```python
from build123d import *

# Parameters (mm, degrees)
AUFSATZ_LINEAR_AUSTRAGEN1_DEPTH      = 20
SCHNITT_LINEAR_AUSTRAGEN1_DEPTH      = 84.102346537
SKIZZE3_R                            = 3.15
SCHNITT_LINEAR_AUSTRAGEN2_DEPTH      = 84.102346537
SCHNITT_LINEAR_AUSTRAGEN3_DEPTH      = 2
SKIZZE5_R                            = 0.75
SCHNITT_LINEAR_AUSTRAGEN4_DEPTH      = 2
SKIZZE6_W                            = 35.5
SKIZZE6_H                            = 6.955295524
AUFSATZ_LINEAR_AUSTRAGEN2_DEPTH      = 20
SKIZZE7_W                            = 7.611739691
SKIZZE7_H                            = 53.192525908
AUFSATZ_LINEAR_AUSTRAGEN3_DEPTH      = 20
SKIZZE8_W                            = 7
SKIZZE8_H                            = 20
AUFSATZ_LINEAR_AUSTRAGEN4_DEPTH      = 27.7
SCHNITT_LINEAR_AUSTRAGEN5_DEPTH      = 26.48
SCHNITT_LINEAR_AUSTRAGEN6_DEPTH      = 6
SCHNITT_LINEAR_AUSTRAGEN6_DEPTH_BACK = 26.48
SKIZZE10_R                           = 1.75
SKIZZE11_R                           = 3
AUFSATZ_LINEAR_AUSTRAGEN5_DEPTH      = 4
SKIZZE12_W                           = 4.692525908
SKIZZE12_H                           = 20
SCHNITT_LINEAR_AUSTRAGEN7_DEPTH      = 130.77615571


with BuildPart() as part:
    # Skizze1 → Aufsatz-Linear austragen1 (new body)
    with BuildSketch(Plane(origin=(0, 0, 0), x_dir=(1, 0, 0), z_dir=(0, 1, 0))):
        with BuildLine():
            Line((0, 59), (0, 0))
            Line((0, 0), (3, 0))
            Line((3, 0), (3, 51.3))
            ThreePointArc((3, 51.3), (4.376598128, 54.623401872), (7.7, 56))
            Line((7.7, 56), (47.3, 56))
            ThreePointArc((47.3, 56), (50.623401872, 54.623401872), (52, 51.3))
            Line((52, 51.3), (52, 0))
            Line((52, 0), (55, 0))
            Line((55, 0), (55, 54.3))
            ThreePointArc((55, 54.3), (53.623401872, 57.623401872), (50.3, 59))
            Line((50.3, 59), (0, 59))
        make_face()
    extrude(amount=AUFSATZ_LINEAR_AUSTRAGEN1_DEPTH)

    # Skizze2 → Schnitt-Linear austragen1 (cut, through all)
    with BuildSketch(Plane(origin=(55, 0, 0), x_dir=(0, 0, -1), z_dir=(1, 0, 0))):
        with BuildLine():
            ThreePointArc((0, 10), (2.928932188, 17.071067812), (10, 20))
            Line((10, 20), (0, 20))
            Line((0, 20), (0, 10))
        make_face()
        with BuildLine():
            ThreePointArc((10, 0), (2.928932188, 2.928932188), (0, 10))
            Line((0, 10), (0, 0))
            Line((0, 0), (10, 0))
        make_face()
    extrude(amount=-SCHNITT_LINEAR_AUSTRAGEN1_DEPTH, mode=Mode.SUBTRACT)

    # Skizze3 → Schnitt-Linear austragen2 (cut, through all)
    with BuildSketch(Plane(origin=(55, 0, 0), x_dir=(0, 0, -1), z_dir=(1, 0, 0))):
        with Locations((10, 10)):
            Circle(SKIZZE3_R)
    extrude(amount=-SCHNITT_LINEAR_AUSTRAGEN2_DEPTH, mode=Mode.SUBTRACT)

    # Skizze4 → Schnitt-Linear austragen3 (cut)
    with BuildSketch(Plane.ZY.offset(-52)):
        with BuildLine():
            Line((-27.5, 7.5), (-12.823894492, 4.145461598))
            ThreePointArc((-12.823894492, 4.145461598), (-3.5, 10), (-12.823894492, 15.854538402))
            Line((-12.823894492, 15.854538402), (-27.5, 12.5))
            ThreePointArc((-27.5, 12.5), (-30, 10), (-27.5, 7.5))
        make_face()
    extrude(amount=-SCHNITT_LINEAR_AUSTRAGEN3_DEPTH, mode=Mode.SUBTRACT)

    # Skizze5 → Schnitt-Linear austragen4 (cut)
    with BuildSketch(Plane.ZY.offset(-54)):
        with Locations((-26.5, 10)):
            Circle(SKIZZE5_R)
        with Locations((-23.5, 10)):
            Circle(SKIZZE5_R)
        with Locations((-20.5, 10)):
            Circle(SKIZZE5_R)
        with Locations((-17.5, 10)):
            Circle(SKIZZE5_R)
    extrude(amount=-SCHNITT_LINEAR_AUSTRAGEN4_DEPTH, mode=Mode.SUBTRACT)

    # Skizze6 → Aufsatz-Linear austragen2 (add)
    with BuildSketch(Plane.XZ):
        with Locations((17.75, -62.477647762)):
            Rectangle(SKIZZE6_W, SKIZZE6_H)
    extrude(amount=-AUFSATZ_LINEAR_AUSTRAGEN2_DEPTH)

    # Skizze7 → Aufsatz-Linear austragen3 (add)
    with BuildSketch(Plane.XZ):
        with Locations((3.805869846, -92.551558478)):
            Rectangle(SKIZZE7_W, SKIZZE7_H)
    extrude(amount=-AUFSATZ_LINEAR_AUSTRAGEN3_DEPTH)

    # Skizze8 → Aufsatz-Linear austragen4 (add)
    with BuildSketch(Plane(origin=(7.611739691, 0, 0), x_dir=(0, 0, -1), z_dir=(1, 0, 0))):
        with Locations((110.955295524, 10)):
            Rectangle(SKIZZE8_W, SKIZZE8_H)
    extrude(amount=AUFSATZ_LINEAR_AUSTRAGEN4_DEPTH)

    # Skizze9 → Schnitt-Linear austragen5 (cut)
    with BuildSketch(Plane(origin=(0, 0, -119.147821432), x_dir=(-1, 0, 0), z_dir=(0, 0, -1))):
        with BuildLine():
            Line((-9.3, 13.5), (-29.794038703, 13.5))
            ThreePointArc((-29.794038703, 13.5), (-31.066830909, 12.972792206), (-31.594038703, 11.7))
            Line((-31.594038703, 11.7), (-31.594038703, 8.3))
            ThreePointArc((-31.594038703, 8.3), (-31.066830909, 7.027207794), (-29.794038703, 6.5))
            Line((-29.794038703, 6.5), (-9.3, 6.5))
            ThreePointArc((-9.3, 6.5), (-8.027207794, 7.027207794), (-7.5, 8.3))
            Line((-7.5, 8.3), (-7.5, 11.7))
            ThreePointArc((-7.5, 11.7), (-8.027207794, 12.972792206), (-9.3, 13.5))
        make_face()
    extrude(amount=-SCHNITT_LINEAR_AUSTRAGEN5_DEPTH, mode=Mode.SUBTRACT)

    # Skizze10 → Schnitt-Linear austragen6 (cut, two sides: drawn at the far end of the back side and taken through both)
    with BuildSketch(Plane(origin=(35.311739691, 0, 0), x_dir=(0, 0, -1), z_dir=(1, 0, 0)).offset(-SCHNITT_LINEAR_AUSTRAGEN6_DEPTH_BACK)):
        with Locations((62.055295524, 15)):
            Circle(SKIZZE10_R)
        with Locations((62.055295524, 5)):
            Circle(SKIZZE10_R)
        with Locations(Location((110.855295524, 5, 0), (0, 0, 180))):
            Circle(SKIZZE10_R)
        with Locations(Location((110.855295524, 15, 0), (0, 0, 180))):
            Circle(SKIZZE10_R)
    extrude(amount=SCHNITT_LINEAR_AUSTRAGEN6_DEPTH + SCHNITT_LINEAR_AUSTRAGEN6_DEPTH_BACK, mode=Mode.SUBTRACT)

    # Skizze11 → Aufsatz-Linear austragen5 (add)
    with BuildSketch(Plane.ZY):
        with Locations((-96.955295524, 10)):
            Circle(SKIZZE11_R)
    extrude(amount=AUFSATZ_LINEAR_AUSTRAGEN5_DEPTH)

    # Skizze12 → Schnitt-Linear austragen7 (cut, through all)
    with BuildSketch(Plane(origin=(7.611739691, 0, 0), x_dir=(0, 0, -1), z_dir=(1, 0, 0))):
        with Locations((116.801558478, 10)):
            Rectangle(SKIZZE12_W, SKIZZE12_H)
    extrude(amount=-SCHNITT_LINEAR_AUSTRAGEN7_DEPTH, mode=Mode.SUBTRACT)


solid = part.part
```
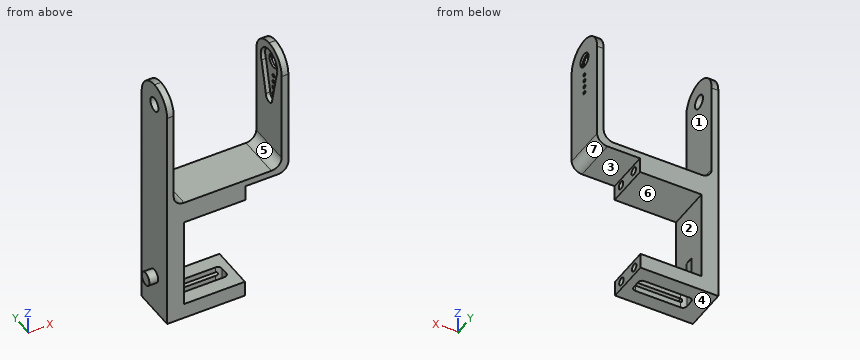
Check sheet for the modelled part. Datum: model origin and axes. Units: mm. Face numbers are marked on the shaded views. A direction names the side the tool comes from. Coordinates: 2 decimals unless noted, no trailing zeros. Order: outer loops, then holes, each group sorted by start corner. A loop starts at its lowest first (then second) coordinate and runs counter-clockwise, first axis right, second up. Notation, with made-up numbers: M 30,-22.5 L 71,-22.5 A20 cw 71,-1.5 Z; hole C 35,-23 d7. An arc over 180 degrees is marked long. Write each question's results on one line, items separated by ' | '. Start each with the question number.
1. Go/stop test with flat-tipped pins: P1, Ø4.5, axis at x = 40, y = 9.5, coming from the -Z side; P2, Ø1, axis at y = 15.5, z = -62, coming from the +X side; P3, Ø1, axis at y = 10, z = -108, coming from the +X side. Record where each tip stops, or that it passes through.
2. Cross-section at B-B on z = -36.5. Record the cut outline in (x, y).
3. Cross-section at C-C on y = 2. Record the cut outline in (x, z), and give its area (3 significant figures).
4. Material ranges on probe 1 along Z at (x, y) = (20, 15); probe 2 along Z at (x, y) = (33.5, 12); probe 3 along X at (y, z) = (15.25, -20), recorded low to high.
5. Cross-section at A-A on x = 16. Record the cut outline in (y, z), and give its area (3 significant figures).
6. Access from +Z, -Z, +X, -X, +Y, -Y to the whole of each face (thin tool, end or side, straight path). Record for the marked faces 1, 2, 3 and 4.
7. Mould release check, pull along X, two halves, no side actions. Record for the marked faces 5, 6 and 7: +X half, -X half, draft (parallel to the pull), parting line (faces both ways), or undercut.
8. Cross-section at D-D on x = 44. Record the cut outline in (y, z), and give its area (3 significant figures).
Checks:
1) P1: stops at z = -59 | P2: stops at x = 8.83 | P3: stops at x = 35.31
2) outline: M 0,0 L 3,0 L 3,20 L 0,20 Z; M 52,0 L 55,0 L 55,20 L 52,20 Z
3) outline: M 0,-114.46 L 35.31,-114.46 L 35.31,-107.46 L 7.61,-107.46 L 7.61,-65.96 L 35.5,-65.96 L 35.5,-59 L 50.3,-59 A4.7 ccw 55,-54.3 L 55,-4 L 52,-4 L 52,-51.3 A4.7 cw 47.3,-56 L 7.7,-56 A4.7 cw 3,-51.3 L 3,-4 L 0,-4 Z | area: 1,290 mm²
4) probe 1: z = -114.46 to -112.61, -109.11 to -107.46, -65.96 to -63.81, -60.31 to -56 | probe 2: z = -114.46 to -107.46, -65.96 to -56 | probe 3: x = 0 to 3, 52 to 55
5) outline: M 0,-114.46 L 6.5,-114.46 L 6.5,-111.76 A1.75 cw long 6.5,-109.95 L 6.5,-107.46 L 0,-107.46 Z; M 0,-65.96 L 20,-65.96 L 20,-56 L 0,-56 Z; M 13.5,-114.46 L 20,-114.46 L 20,-107.46 L 13.5,-107.46 L 13.5,-109.95 A1.75 cw long 13.5,-111.76 Z; hole C 5,-62.06 d3.5; hole C 15,-62.06 d3.5 | area: 252 mm²
6) face 1: +Z, +Y, -Y | face 2: +X, +Y, -Y | face 3: -Z, +X, +Y, -Y | face 4: -Z, +X, -X, +Y, -Y
7) face 5: undercut | face 6: draft | face 7: +X half
8) outline: M 0,-59 L 20,-59 L 20,-56 L 0,-56 Z | area: 60.0 mm²
